Part print with two shaded views. Sizes in mm from the minimum x, y, z corner. Coordinates: 2 decimals unless noted, no trailing zeros. Order: outer loops, then holes, each group sorted by start corner. A loop starts at its lowest first (then second) coordinate and runs counter-clockwise, first axis right, second up. Notation, with made-up numbers: (-36, 1) - (-13, 1) arc R21 ccw to (-13, 25) - close; hole circle Ø8 at (-8.75, 27.5). An arc over 180 degrees is marked (long way). Write each question's results on one line, items separated by ' | '. Start each with the question number.
Q1. Pull direction X, two halves, no side cores. Call the marked faces 1, 2 and 3: released by +X, released by -X, zero draft, split by the parting line, or undercut.
Q2. Band-saw the part on A-A, the plane z = 1.75. Write the cut outline in (x, y), then the cut area to 3 significant figures.
Q3. Pin check, flat tips, straight feed: P1, Ø1.5, axis at x = 5.5, z = 0.5, coming from the -Y side; P2, Ø4, axis at x = 5, y = 4, coming from the -Z side; P3, Ø3, axis at x = 6, z = 2, coming from the +Y side. Stop position of each tip, or through.
Q4. Wall check: probe 1 along X at (y, z) = (6.5, 3.7) (1 decimal); probe 2 along X at (y, z) = (4.75, 4.45); probe 3 along Y at (x, z) = (5.5, 2.6) (1 decimal). Give the ranges that are in metal, low to high.
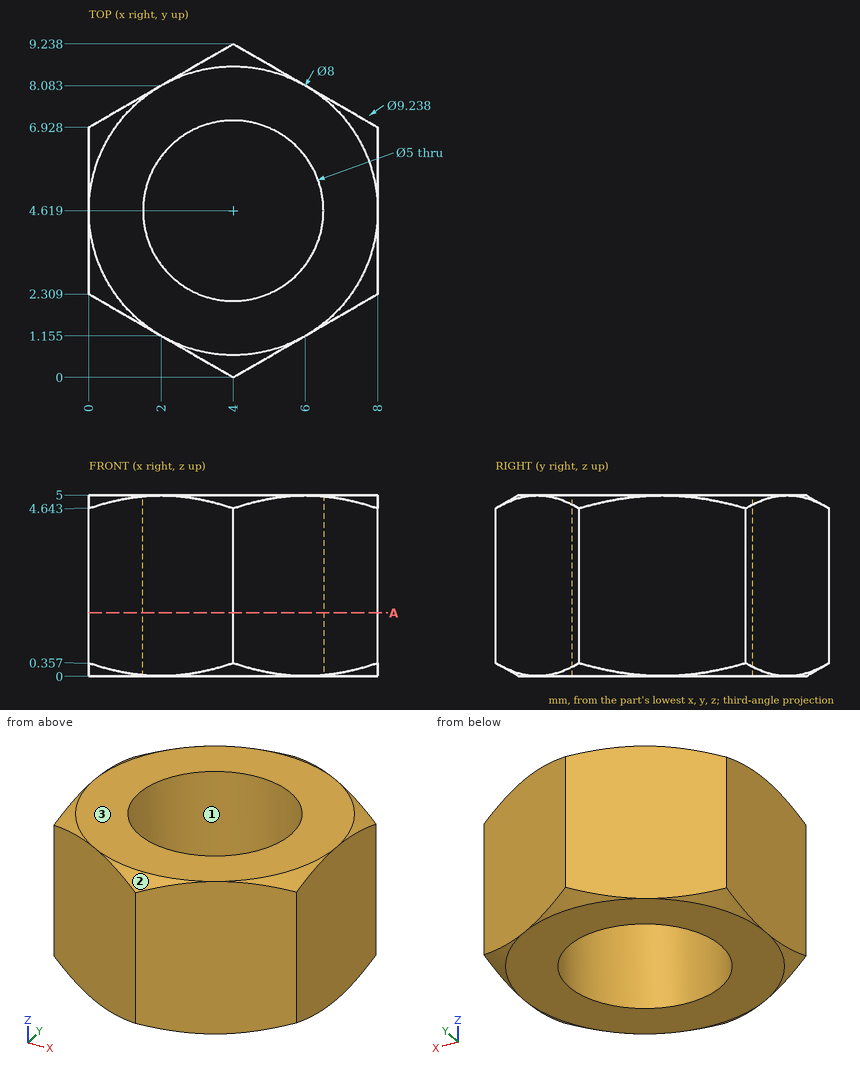
Results below:
1) face 1: undercut | face 2: split by the parting line | face 3: zero draft
2) outline: (0, 2.31) - (4, 0) - (8, 2.31) - (8, 6.93) - (4, 9.24) - (0, 6.93) - close; hole circle Ø5 at (4, 4.62) | area: 35.8 mm²
3) P1: stops at y = 0.43 | P2: stops at z = 0 | P3: stops at y = 8.95
4) probe 1: x = 0 to 2.4, 5.6 to 8 | probe 2: x = 0 to 1.5, 6.5 to 8 | probe 3: y = 0.9 to 2.6, 6.6 to 8.4
